```python
from build123d import *

# Parameters (mm, degrees)
SKETCH_1_W          = 37
SKETCH_1_H          = 10
EXTRUDE_1_DEPTH     = 7.25
EXTRUDE_2_DEPTH     = 4
FILLET_1_R          = 5
CUT_EXTRUDE_1_DEPTH = 3
CUT_EXTRUDE_3_DEPTH = 4
HOLE_WIZARD_M3_1_D  = 2.5
SKETCH_7_W          = 20.003423604
SKETCH_7_H          = 10
EXTRUDE_3_DEPTH     = 22.75
SKETCH_8_R          = 3
EXTRUDE_4_DEPTH     = 8
FILLET_2_R          = 2


with BuildPart() as part:
    # 草图1 → 凸台-拉伸1 (new body)
    with BuildSketch(Plane(origin=(0, 0, 0), x_dir=(1, 0, 0), z_dir=(0, 1, 0))):
        Rectangle(SKETCH_1_W, SKETCH_1_H)
    extrude(amount=EXTRUDE_1_DEPTH)

    # 草图2 → 凸台-拉伸2 (add)
    with BuildSketch(Plane(origin=(0, 7.25, 0), x_dir=(1, 0, 0), z_dir=(0, 1, 0))):
        Polygon((-8.75, 0), (-5.75, 3), (5.75, 3), (8.75, 0), (8.75, -3), (-8.75, -3), align=None)
    extrude(amount=EXTRUDE_2_DEPTH)

    # 圆角1
    fillet_1_edges = [part.edges().sort_by_distance(p)[0] for p in [
        (18.5, 3.625, 5),
        (18.5, 3.625, -5),
        (-18.5, 3.625, 5),
        (-18.5, 3.625, -5),
    ]]
    fillet(fillet_1_edges, radius=FILLET_1_R - 0.0001)  # a hair under: the kernel refuses the full size

    # 草图3 → 切除-拉伸1 (cut)
    with BuildSketch(Plane(origin=(0, 11.25, 0), x_dir=(1, 0, 0), z_dir=(0, 1, 0))):
        Polygon((8.75, -3), (8.75, 0), (5.75, 3), (-5.75, 3), (-8.75, 0), (-8.75, -3), align=None)
        Polygon((7.75, -2), (7.75, -0.414213562), (5.335786438, 2), (-5.335786438, 2), (-7.75, -0.414213562), (-7.75, -2), align=None, mode=Mode.SUBTRACT)
    extrude(amount=-CUT_EXTRUDE_1_DEPTH, mode=Mode.SUBTRACT)

    # 草图4 → 切除-拉伸3 (cut)
    with BuildSketch(Plane(origin=(0, 11.25, 0), x_dir=(1, 0, 0), z_dir=(0, 1, 0))):
        Polygon((-7.55, -0.497056275), (-7.55, -1.8), (7.55, -1.8), (7.55, -0.497056275), (5.252943725, 1.8), (-5.252943725, 1.8), align=None)
    extrude(amount=-CUT_EXTRUDE_3_DEPTH, mode=Mode.SUBTRACT)

    # M3 螺纹孔1 (through all)
    with Locations(Plane(origin=(0, 7.25, 0), x_dir=(1, 0, 0), z_dir=(0, 1, 0))):
        with Locations((-13.5, 0), (13.5, 0)):
            Hole(HOLE_WIZARD_M3_1_D / 2)

    # 草图7 → 凸台-拉伸3 (add)
    with BuildSketch(Plane.XZ):
        Rectangle(SKETCH_7_W, SKETCH_7_H)
    extrude(amount=EXTRUDE_3_DEPTH)

    # 草图8 → 凸台-拉伸4 (add)
    with BuildSketch(Plane.XZ.offset(22.75)):
        with Locations(Location((0, 0, 0), (0, 0, 270))):
            Circle(SKETCH_8_R)
    extrude(amount=EXTRUDE_4_DEPTH)

    # 圆角2
    fillet_2_edges = [part.edges().sort_by_distance(p)[0] for p in [
        (-10.001711802, -11.375, 5),
        (-10.001711802, -11.375, -5),
        (10.001711802, -11.375, -5),
        (10.001711802, -11.375, 5),
        (-10.001711802, -22.75, 0),
        (0, -22.75, -5),
        (10.001711802, -22.75, 0),
        (0, -22.75, 5),
    ]]
    fillet(fillet_2_edges, radius=FILLET_2_R - 0.0001)  # a hair under: the kernel refuses the full size


solid = part.part
```
Geometry: final body of the model. Coordinates: model frame, mm. A direction names the side the tool comes from. Round coordinates to 2 decimals unless told otherwise and drop trailing zeros. Write each loop counter-clockwise with the first axis right and the second up, starting at its lowest first coordinate (ties: lowest second). Pieces come first, ordered by that corner, then holes.
Item 1: Mould query, pull axis Z, two halves, no side actions, for faces 1 (the face through (6.56, 9.771, -0.776)), 2 (the face through (10.002, -10, 0)), 3 (the face through (17, 3.68, 3.57)), 4 (the face through (-12.25, 3.57, -0.05)). Classes: +Z half, -Z half, draft (parallel to the pull), parting line (faces both ways), or undercut.
Item 2: Material intervals for L1, parallel to Z at x = -13.5, y = 3.5; L2, parallel to Y at x = -16, z = 1; L3, parallel to Y at x = -7, z = -2.25, sorted ascending.
Item 3: Section query C-C (y = -7.5). Return loops of the section in (x, z).
Item 4: Pin query (flat end, axial travel): P1, Ø0.8, axis at y = 8, z = 1, coming from the -X side; P2, Ø4, axis at x = -4.5, z = 2.5, coming from the -Y side; P3, Ø2, axis at x = -13.5, z = 0, coming from the -Y side; P4, Ø1, axis at y = 9.5, z = 1, coming from the +X side. Return the tip coordinate at first contact, or that it passes through.
Item 5: Section query D-D (z = 4). Return loops of the section in (x, y).
Item 6: Section query A-A (z = -0.5). Give the number of separate pieces and of enclosed holes in the cut face, plus the area to 3 significant figures.
Item 7: Set-up query: faces 5 (the face through (0, 9, 1.8)), 6 (the face through (0, 10, -2)), 7 (the face through (-9.4, -10.52, -4.43)), 8 (the face through (-8.75, 8, 2)), 9 (the face through (0, 8, 3)). Return all of +Z, -Z, +X, -X, +Y, -Y with unobstructed straight access to the full face (end or side cutting, diameter ignored); none if empty.
Completed:
1. face 1: -Z half
1. face 2: draft
1. face 3: +Z half
1. face 4: undercut
2. L1: z = -5 to -1.25, 1.25 to 5
2. L2: y = 0 to 7.25
2. L3: y = -22.75 to 7.25
3. outline: (-10, -3) arc R2 ccw to (-8, -5) - (8, -5) arc R2 ccw to (10, -3) - (10, 3) arc R2 ccw to (8, 5) - (-8, 5) arc R2 ccw to (-10, 3) - close
4. P1: stops at x = -8.75
4. P2: stops at y = -22.75
4. P3: passes through
4. P4: stops at x = 7.75
5. outline: (-16.5, 0) - (-9.73, 0) - (-9.73, -20.75) arc R1.73 ccw to (-8, -22.48) - (8, -22.48) arc R1.73 ccw to (9.73, -20.75) - (9.73, 0) - (16.5, 0) - (16.5, 7.25) - (-16.5, 7.25) - close
6. separate pieces: 3
6. enclosed holes: 0
6. area: 740 mm2
7. face 5: +Y
7. face 6: -Z, +X, -X, +Y
7. face 7: -Z, -X, -Y
7. face 8: +Z, -Z, -X, +Y
7. face 9: +Z, +X, -X, +Y
